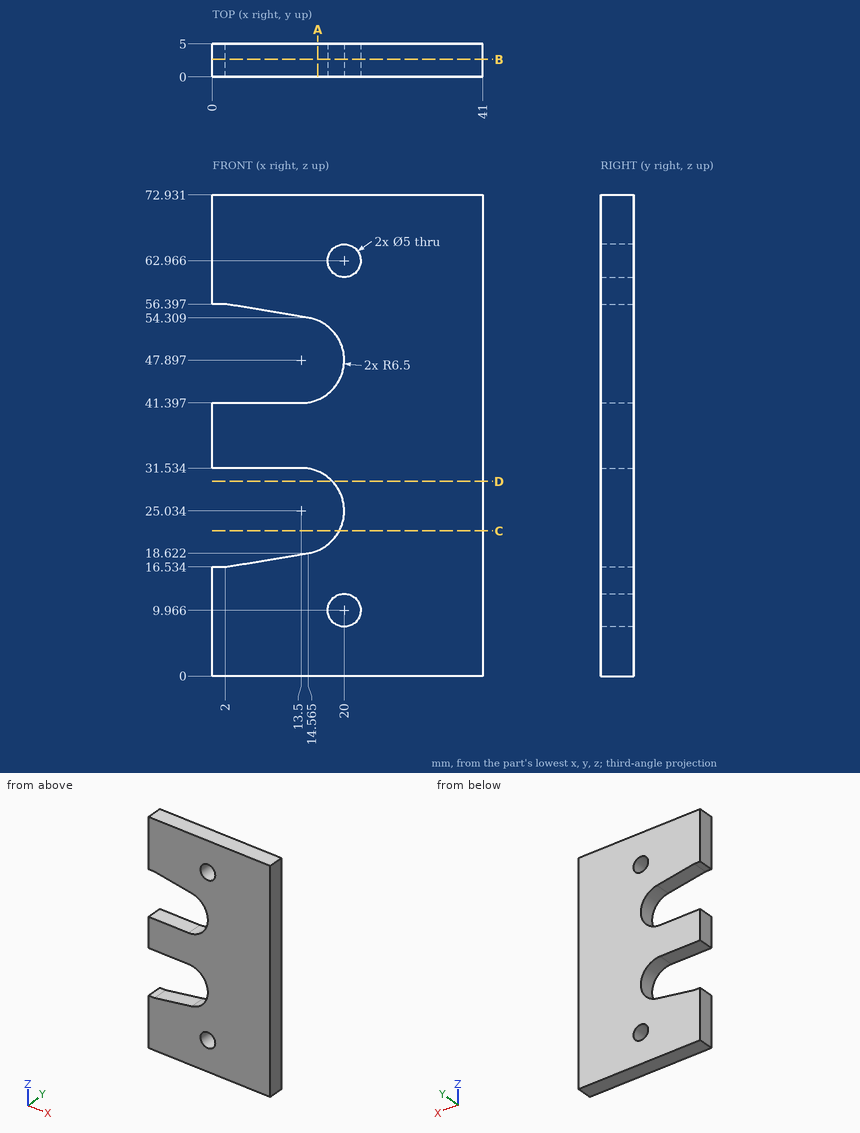
The figure shows three views and two pictorial views of one solid part (mm, origin at its lowest corner). Answer the questions. Give positions to 0.01 mm unless a question says otherwise; leave off trailing zeros. Write each loop counter-clockwise with the first axis right and the second up, starting at its lowest first coordinate (ties: lowest second). Pieces come first, ordered by that corner, then holes.
Q1. The part is cut by section C-C on z = 22. Give the vertices of the cut face in (x, y), and give its area (3 significant figures).
Answer:
outline: (19.25, 0) - (41, 0) - (41, 5) - (19.25, 5) - close
area: 109 mm2
Q2. Given pin 1 (1.5 mm diameter, centred on y = 1, z = 32.5, fed in from -X), flat-ended and moving along its own axis, determine where the tip first touches the part or whether it passes through.
Answer:
pin 1: stops at x = 0
Q3. The part is cut by section D-D on z = 29.5. Give the vertices of the cut face in (x, y).
Answer:
outline: (18.22, 0) - (41, 0) - (41, 5) - (18.22, 5) - close
Q4. Straight lines are drawn through the part: L1, parallel to Z at x = 13, y = 4.2 (1 decimal); L2, parallel to Z at x = 7, y = 2.35 (1 decimal); L3, parallel to X at y = 2.95, z = 45. For each, find the intervals that lie inside material, in ascending order.
Answer:
L1: z = 0 to 18.4, 31.5 to 41.4, 54.6 to 72.9
L2: z = 0 to 17.4, 31.5 to 41.4, 55.6 to 72.9
L3: x = 19.32 to 41
Q5. The part is cut by section B-B on y = 2.65. Give the vertices of the cut face in (x, z) (1 decimal), and give its area (4 significant figures).
Answer:
outline: (0, 0) - (41, 0) - (41, 72.9) - (0, 72.9) - (0, 56.4) - (2, 56.4) - (14.6, 54.3) arc R6.5 cw to (13.5, 41.4) - (0, 41.4) - (0, 31.5) - (13.5, 31.5) arc R6.5 cw to (14.6, 18.6) - (2, 16.5) - (0, 16.5) - close; hole circle Ø5 at (20, 10); hole circle Ø5 at (20, 63)
area: 2,435 mm2
Q6. The part is cut by section A-A on x = 16. Give the vertices of the cut face in (y, z) (1 decimal).
Answer:
outline: (0, 0) - (5, 0) - (5, 19) - (0, 19) - close; (0, 31) - (5, 31) - (5, 41.9) - (0, 41.9) - close; (0, 53.9) - (5, 53.9) - (5, 72.9) - (0, 72.9) - close
